```python
from build123d import *

# Parameters (mm, degrees)
F0_W     = 750
F0_H     = 400
F1_DEPTH = 20
F2_W     = 20
F2_H     = 50
F2_H_2   = 30
F3_DEPTH = 20
F2_H_3   = 20
F2_W_2   = 30
F2_W_3   = 50
F4_DEPTH = 20


with BuildPart() as f1:
    # F0 (on Front) → F1 (new body)
    with BuildSketch(Plane.XZ):
        with Locations((4.104346, -200)):
            Rectangle(F0_W, F0_H)
    extrude(amount=F1_DEPTH)

    # F2 (on face) → F3 (cut)
    with BuildSketch(Plane.XZ.offset(20)):
        with Locations((-360.895654, -25)):
            Rectangle(F2_W, F2_H)
        with Locations((-360.895654, -125)):
            Rectangle(F2_W, F2_H)
        with Locations((-360.895654, -225)):
            Rectangle(F2_W, F2_H)
        with Locations((-360.895654, -325)):
            Rectangle(F2_W, F2_H)
        with Locations((369.104346, -365)):
            Rectangle(F2_W, F2_H_2)
        with Locations((369.104346, -275)):
            Rectangle(F2_W, F2_H)
        with Locations((369.104346, -175)):
            Rectangle(F2_W, F2_H)
        with Locations((369.104346, -75)):
            Rectangle(F2_W, F2_H)
    extrude(amount=-F3_DEPTH, mode=Mode.SUBTRACT)

    # F2 (on face) → F4 (cut)
    with BuildSketch(Plane.XZ.offset(20)):
        with Locations((-360.895654, -390)):
            Rectangle(F2_W, F2_H_3)
        with Locations((-335.895654, -390)):
            Rectangle(F2_W_2, F2_H_3)
        with Locations((-245.895654, -390)):
            Rectangle(F2_W_3, F2_H_3)
        with Locations((-145.895654, -390)):
            Rectangle(F2_W_3, F2_H_3)
        with Locations((-45.895654, -390)):
            Rectangle(F2_W_3, F2_H_3)
        with Locations((54.104346, -390)):
            Rectangle(F2_W_3, F2_H_3)
        with Locations((154.104346, -390)):
            Rectangle(F2_W_3, F2_H_3)
        with Locations((254.104346, -390)):
            Rectangle(F2_W_3, F2_H_3)
        with Locations((344.104346, -390)):
            Rectangle(F2_W_2, F2_H_3)
        with Locations((369.104346, -390)):
            Rectangle(F2_W, F2_H_3)
    extrude(amount=-F4_DEPTH, mode=Mode.SUBTRACT)


solid = f1.part
```
Work out the finished part from the listing and answer in its coordinate system (mm). A direction names the side the tool comes from. Give positions to 0.01 mm unless a question says otherwise; leave off trailing zeros. Loops run counter-clockwise (first coordinate to the right, second up) from the corner with the lowest first, then second, coordinate; pieces in that order, holes last. Notation, with made-up numbers: M 86,4.5 L 99,4.5 A8 ccw 99,10.5 Z; hole C -32,81 d4. An arc over 180 degrees is marked long. One line per item, written item: value. Start each with the question number.
1. Find section A-A (z = -341). Give the vertices of the cut face in (x, y), and give its area (3 significant figures).
2. Determine the mould class of faces 1 (the face through (-346, -10, -380)), 2 (the face through (-350.896, -10, -125)), 3 (the face through (-246, -10, -380)) for opening direction X: released by +X, released by -X, zero draft, split by the parting line, or undercut.
3. Find section B-B (x = -137.5). Give the vertices of the cut face in (y, z).
4. Each of these flat-tipped pins is pushed along its axis until it touches: P1, Ø1.5, axis at y = -10.5, z = -130.5, coming from the -X side; P2, Ø6, axis at x = 54.5, y = -11.5, coming from the -Z side; P3, Ø6, axis at y = -9.5, z = -392.5, coming from the +X side. Where does it stop, or does it pass through?
5. Find the intervals of material crossed by probe 1 along X at (y, z) = (-3, -313.5); probe 2 along Z at (x, y) = (-236, -14.5); probe 3 along X at (y, z) = (-16.25, -178), in increasing order.
6. Which of the six approach directions +Z, -Z, +X, -X, +Y, -Y give full straight-line access (tool end or side, diameter ignored) to faces 4 (the face through (-1, -20, -197)), 5 (the face through (-46, -10, -380)), 6 (the face through (359.104, -10, -75)), 7 (the face through (-350.896, -10, -225)), 8 (the face through (9, -10, 0))?
Reported:
1. outline: M -350.9,-20 L 379.1,-20 L 379.1,0 L -350.9,0 Z
1. area: 14,600 mm²
2. face 1: zero draft
2. face 2: released by -X
2. face 3: undercut
3. outline: M -20,-380 L 0,-380 L 0,0 L -20,0 Z
4. P1: stops at x = -350.9
4. P2: stops at z = -380
4. P3: stops at x = 329.1
5. probe 1: x = -350.9 to 379.1
5. probe 2: z = -380 to 0
5. probe 3: x = -370.9 to 359.1
6. face 4: +Z, -Z, +X, -X, -Y
6. face 5: -Z, +Y, -Y
6. face 6: +X, +Y, -Y
6. face 7: -X, +Y, -Y
6. face 8: +Z, +X, -X, +Y, -Y
